from build123d import *

# Parameters (mm, degrees)
BOSS_EXTRUDE1_DEPTH     = 50
BOSS_EXTRUDE2_DEPTH     = 55
BOSS_EXTRUDE3_DEPTH     = 27.5
CUT_EXTRUDE1_DEPTH      = 20
CUT_EXTRUDE2_DEPTH      = 434.416658655
CUT_EXTRUDE2_DEPTH_BACK = 434.416658655
CUT_EXTRUDE3_DEPTH      = 444.762323773
CUT_EXTRUDE3_DEPTH_BACK = 444.762323773
SKETCH6_W               = 10
SKETCH6_H               = 90
SKETCH7_R               = 25
BOSS_EXTRUDE4_DEPTH     = 5
LPATTERN1_COUNT         = 2
LPATTERN1_PITCH         = 290
HOLE1_D                 = 20
HOLE2_D                 = 16
HOLE2_DEPTH             = 25
LPATTERN2_COUNT         = 2
LPATTERN2_PITCH         = 140
FILLET1_R               = 25
FILLET2_R               = 13
FILLET3_R               = 20
FILLET4_R               = 10


with BuildPart() as part:
    # Sketch1 → Boss-Extrude1 (new, symmetric)
    with BuildSketch(Plane(origin=(0, 0, 0), x_dir=(0, 0, -1), z_dir=(1, 0, 0))):
        Polygon((0, 0), (0, 30), (100, 30), (100, 235), (125, 235), (125, 30), (360, 30), (360, 0), align=None)
    extrude(amount=BOSS_EXTRUDE1_DEPTH, both=True)

    # Sketch2 → Boss-Extrude2 (add, symmetric)
    with BuildSketch(Plane(origin=(0, 0, 0), x_dir=(0, 0, -1), z_dir=(1, 0, 0))):
        with BuildLine():
            Line((100, 195), (100, 95))
            ThreePointArc((100, 95), (150, 145), (100, 195))
        make_face()
    extrude(amount=BOSS_EXTRUDE2_DEPTH, both=True)

    # Sketch3 → Boss-Extrude3 (add, symmetric)
    with BuildSketch(Plane(origin=(0, 0, 0), x_dir=(0, 0, -1), z_dir=(1, 0, 0))):
        with BuildLine():
            Line((125, 235), (125, 30))
            Line((125, 30), (262.632576463, 30))
            Line((262.632576463, 30), (209.572335871, 175.781812899))
            ThreePointArc((209.572335871, 175.781812899), (176.621879272, 218.723683986), (125, 235))
        make_face()
    extrude(amount=BOSS_EXTRUDE3_DEPTH, both=True)

    # Sketch4 → Cut-Extrude1 (cut)
    with BuildSketch(Plane(origin=(27.5, 0, 0), x_dir=(0, 0, -1), z_dir=(1, 0, 0))):
        with BuildLine():
            Line((125, 225), (125, 188.301270189))
            ThreePointArc((125, 188.301270189), (150, 145), (125, 101.698729811))
            Line((125, 101.698729811), (125, 30))
            Line((125, 30), (251.990798739, 30))
            Line((251.990798739, 30), (200.175409663, 172.361611466))
            ThreePointArc((200.175409663, 172.361611466), (170.886114908, 210.532163543), (125, 225))
        make_face()
    cut_extrude1 = extrude(amount=-CUT_EXTRUDE1_DEPTH, mode=Mode.SUBTRACT)

    # Mirror1: Cut-Extrude1 across plane
    add(cut_extrude1.mirror(Plane(origin=(0, 0, 0), x_dir=(0, 0, 1), z_dir=(1, 0, 0))), mode=Mode.SUBTRACT)

    # Sketch5 → Cut-Extrude2 (cut, two sides: drawn at the far end of the back side and taken through both)
    with BuildSketch(Plane(origin=(0, 0, 0), x_dir=(0, 0, -1), z_dir=(1, 0, 0)).offset(-CUT_EXTRUDE2_DEPTH_BACK)):
        with BuildLine():
            Line((100, 185), (100, 105))
            ThreePointArc((100, 105), (140, 145), (100, 185))
        make_face()
    extrude(amount=CUT_EXTRUDE2_DEPTH + CUT_EXTRUDE2_DEPTH_BACK, mode=Mode.SUBTRACT)

    # Sketch6 → Cut-Extrude3 (cut, two sides: drawn at the far end of the back side and taken through both)
    with BuildSketch(Plane(origin=(55, 0, 0), x_dir=(0, 0, -1), z_dir=(1, 0, 0)).offset(-CUT_EXTRUDE3_DEPTH_BACK)):
        with Locations((100, 145)):
            Rectangle(SKETCH6_W, SKETCH6_H)
    extrude(amount=CUT_EXTRUDE3_DEPTH + CUT_EXTRUDE3_DEPTH_BACK, mode=Mode.SUBTRACT)

    # Sketch7 → Boss-Extrude4 (add)
    with BuildSketch(Plane(origin=(0, 30, 0), x_dir=(1, 0, 0), z_dir=(0, 1, 0))):
        with Locations(Location((0, 35, 0), (0, 0, 90))):
            Circle(SKETCH7_R)
    boss_extrude4 = extrude(amount=BOSS_EXTRUDE4_DEPTH)

    # LPattern1: Boss-Extrude4 ×2
    with Locations(*[(0, 0, -i * LPATTERN1_PITCH) for i in range(1, LPATTERN1_COUNT)]):
        add(boss_extrude4)

    # Hole1 (through all)
    with Locations(Plane(origin=(0, 35, 0), x_dir=(1, 0, 0), z_dir=(0, 1, 0))):
        with Locations((0, 35), (0, 325)):
            Hole(HOLE1_D / 2)

    # Hole2
    with Locations(Plane.XY.offset(-100)):
        with Locations((0, 215)):
            hole2 = Hole(HOLE2_D / 2, depth=HOLE2_DEPTH)

    # LPattern2: Hole2 ×2
    with Locations(*[(0, -i * LPATTERN2_PITCH, 0) for i in range(1, LPATTERN2_COUNT)]):
        add(hole2, mode=Mode.SUBTRACT)

    # Fillet1
    fillet1_edges = [part.edges().sort_by_distance(p)[0] for p in [
        (0, 30, -262.632576463),
    ]]
    fillet(fillet1_edges, radius=FILLET1_R)

    # Fillet2
    fillet2_edges = [part.edges().sort_by_distance(p)[0] for p in [
        (28.75, 30, -125),
        (-28.75, 30, -125),
        (17.5, 30, -251.990798739),
        (-17.5, 30, -251.990798739),
    ]]
    fillet(fillet2_edges, radius=FILLET2_R)

    # Fillet3
    fillet3_edges = [part.edges().sort_by_distance(p)[0] for p in [
        (0, 30, -100),
    ]]
    fillet(fillet3_edges, radius=FILLET3_R)

    # Fillet4
    # the kernel refuses this fillet: 10 mm, written as the material it adds along each edge
    with BuildSketch(Plane(origin=(27.5, 225, -125), x_dir=(0, -1, 0), z_dir=(-1, 0, 0))) as fillet4_piece_1:
        with BuildLine():
            CenterArc((10.717967697, -10), FILLET4_R, 90, 98.213210702)
            ThreePointArc((0.820534511, -11.428571429), (0.205397303, -5.728994715), (0, 0))
            Line((0, 0), (10.717967697, 0))
        make_face()
    extrude(amount=48.644973575)
    with BuildSketch(Plane(origin=(-27.5, 225, -125), x_dir=(0, -1, 0), z_dir=(1, 0, 0))) as fillet4_piece_2:
        with BuildLine():
            CenterArc((10.717967697, 10), FILLET4_R, 171.786789298, 98.213210702)
            ThreePointArc((0.820534511, 11.428571429), (0.205397303, 5.728994715), (0, 0))
            Line((0, 0), (10.717967697, 0))
        make_face()
    extrude(amount=48.644973575)


solid = part.part
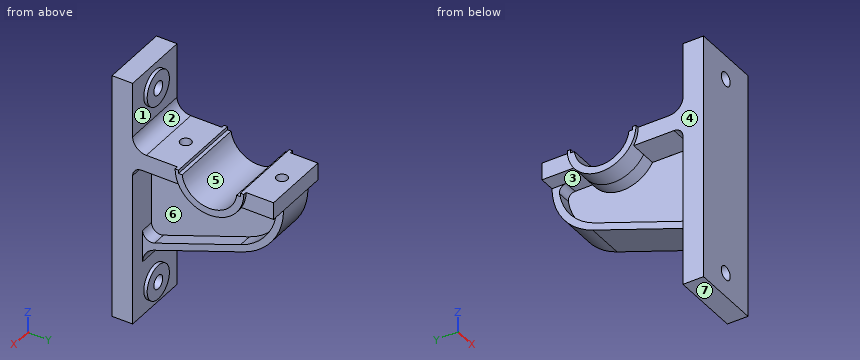
Here's how the part is built. I have some questions about the finished solid (model axes, mm). Face numbers are marked on the shaded views. A direction names the side the tool comes from. Coordinates: 2 decimals unless noted, no trailing zeros. Order: outer loops, then holes, each group sorted by start corner. A loop starts at its lowest first (then second) coordinate and runs counter-clockwise, first axis right, second up. Notation, with made-up numbers: (2, 85.25) -> (23, 85.25) arc R21 cw to (23, 96.25) -> close; hole circle Ø4 at (53.5, -34). An arc over 180 degrees is marked (long way). Answer in a Markdown table with one row per item.
(1) Will these pins go through, and if not, where does the flat tip stop? pin 1 Ø14.5 at (x, y) = (0, 215) entering from -Z; pin 2 Ø13 at (x, y) = (-33, 202) entering from -Z; pin 3 Ø12.5 at (y, z) = (204.5, -113) entering from +X.
Answer key:
| item | result |
|---|---|
| pin 1 | z = -189.52 |
| pin 2 | z = -197.35 |
| pin 3 | x = 50 |
(2) On a 3-axis mill with a long thin cutter (end or side, diameter ignored), from which of +Z, -Z, +X, -X, +Y, -Y can I reach the whole of each face in a straight line? I mean the marked faces 1, 2 and 3. Say none if no direction works.
Answer key:
| item | result |
|---|---|
| face 1 | +Y |
| face 2 | +X, -X, +Y |
| face 3 | -X |
(3) I want a section at A-A on z = -325. List the corners of the cut face in (x, y) for me.
Answer key:
| item | result |
|---|---|
| outline | (-50, 0) -> (-10, 0) -> (-10, 35) -> (-25, 35) -> (-25, 30) -> (-50, 30) -> close; (10, 0) -> (50, 0) -> (50, 30) -> (25, 30) -> (25, 35) -> (10, 35) -> close |
(4) I want a section at C-C on x = -42.5. List the corners of the cut face in (y, z) for me.
Answer key:
| item | result |
|---|---|
| outline | (0, -360) -> (30, -360) -> (30, -138) arc R13 cw to (43, -125) -> (101.7, -125) arc R50 ccw to (188.3, -125) -> (235, -125) -> (235, -100) -> (190, -100) -> (190, -105) -> (184.69, -105) arc R40 cw to (105.31, -105) -> (100, -105) -> (100, -100) -> (50, -100) arc R20 cw to (30, -80) -> (30, 0) -> (0, 0) -> close |
(5) Please list where these lines run through material, in increasing order: probe 1 along Z at (x, y) = (0, 15); probe 2 along Y at (x, z) = (0, -105.25); probe 3 along X at (y, z) = (75, -119).
Answer key:
| item | result |
|---|---|
| probe 1 | -360 to -335, -315 to -45, -25 to 0 |
| probe 2 | 0 to 67, 83 to 105.35, 184.65 to 207, 223 to 235 |
| probe 3 | -50 to -8, 8 to 50 |
(6) I want a section at D-D on x = 0. Count the separate pieces of the cut face and the enclosed holes in it, then the cut area to 3 significant figures.
Answer key:
| item | result |
|---|---|
| separate pieces | 3 |
| enclosed holes | 0 |
| area | 31,600 mm^2 |
(7) Thinking about a two-plate mould opening in Z: for the marked faces 4, 5, 6 and 7, which applies, +Z half, -Z half, draft (parallel to the pull), parting line (faces both ways), or undercut?
Answer key:
| item | result |
|---|---|
| face 4 | draft |
| face 5 | +Z half |
| face 6 | undercut |
| face 7 | -Z half |
